CAD build for the part. Positions are in the model's coordinates, mm. Round coordinates to 2 decimals unless told otherwise and drop trailing zeros. Write each loop counter-clockwise with the first axis right and the second up, starting at its lowest first coordinate (ties: lowest second). Pieces come first, ordered by that corner, then holes. Notation, with made-up numbers: (78, -21) - (126, -21) arc R32 cw to (126, 7) - close; hole circle Ø1 at (50, -25.75). An arc over 180 degrees is marked (long way). Answer in a Markdown table with one row per item.
```python
from build123d import *

# Parameters (mm, degrees)
F0_W      = 128.7249475718
F0_H      = 25.9889103472
F5_DEPTH  = 25.4
F8_DEPTH  = 25.4
F9_DEPTH  = 83.0614138395
F11_DEPTH = 108.5182130337


with BuildPart() as f5:
    # F0 (on Front) → F5 (new body)
    with BuildSketch(Plane.XZ):
        with Locations((64.3624737859, 12.9944551736)):
            Rectangle(F0_W, F0_H)
    extrude(amount=F5_DEPTH)

    # F6 (on Front) + F7 (on face) → F8 (join)
    with BuildSketch(Plane.XZ):
        Polygon((185.9581768513, 0), (128.5665184259, 25.8846282959), (160.3146493435, 0), align=None)
        Polygon((160.3146493435, 0), (128.5665184259, 25.8846282959), (127.9721856117, 0), align=None)
    with BuildSketch(Plane.XZ):
        Polygon((200.6603479385, 0), (138.9337457069, 21.2088298961), (185.9581768513, 0), align=None)
    extrude(amount=F8_DEPTH)

    # F9 (add): a face of the model
    f9_faces = [f5.faces().sort_by_distance(p)[0] for p in [
        (82.97421567, -25.4, 12.0117681363),
    ]]
    extrude(f9_faces, amount=F9_DEPTH)

    # F10 (on Front) → F11 (join)
    with BuildSketch(Plane.XZ):
        Polygon((0, 0), (0, 25.0786654651), (-61.9297772646, 0), align=None)
    extrude(amount=F11_DEPTH)


solid = f5.part
```
Q1. Saw through at C-C on x = -39. List the corners of the cut face in (y, z), then the cut area to 3 significant figures.
Computed:
| item | result |
|---|---|
| outline | (-108.52, 0) - (0, 0) - (0, 9.29) - (-108.52, 9.29) - close |
| area | 1,010 mm2 |
Q2. Drill centre lines: line 1 (Y direction, x = 20.5, z = 7.25); line 2 (Z direction, x = -48.5, y = -22); line 3 (X direction, y = -66, z = 24.75). Where is each one in solid material? Low to high.
Computed:
| item | result |
|---|---|
| line 1 | y = -108.46 to 0 |
| line 2 | z = 0 to 5.44 |
| line 3 | x = -0.81 to 131.08 |
Q3. Saw through at A-A on y = -36.5. List the corners of the cut face in (x, z), then the cut area to 3 significant figures.
Computed:
| item | result |
|---|---|
| outline | (-61.93, 0) - (200.66, 0) - (138.93, 21.21) - (128.72, 25.81) - (128.72, 25.99) - (0, 25.99) - (0, 25.08) - close |
| area | 5,020 mm2 |
Q4. Saw through at B-B on z = 8.75. List the corners of the cut face in (x, y).
Computed:
| item | result |
|---|---|
| outline | (-40.32, -108.52) - (0, -108.52) - (0, -108.46) - (175.19, -108.46) - (175.19, 0) - (-40.32, 0) - close |
Q5. Flat gauge pins, fed straight in: pin 1 (2 mm diameter, centred on y = -62, z = 11.5, fed in from -X); pin 2 (2 mm diameter, centred on x = 155, y = -13.5, fed in from -Z); pin 3 (12 mm diameter, centred on y = -25, z = 13.5, fed in from -X); pin 4 (1 mm diameter, centred on y = -13, z = 23, fed in from -X). Where does each tip first touch, or does it go through?
Computed:
| item | result |
|---|---|
| pin 1 | stops at x = -36 |
| pin 2 | stops at z = 0 |
| pin 3 | stops at x = -43.41 |
| pin 4 | stops at x = -6.37 |
